Solid Edge part; units mm, degrees
sketch "Sketch1" plane through (0, 0, 0) normal (0, 0, 1) x (1, 0, 0)
  line L0 (-15, 5.75) -> (15, 5.75)
  line L1 (15, 5.75) -> (15, -5.75)
  line L2 (15, -5.75) -> (-15, -5.75)
  line L3 (-15, -5.75) -> (-15, 5.75)
  dimension "D1" = 15
  dimension "D2" = 15
extrude "Protrusion1" add sketch "Sketch1" along normal blind 3
fillet "Avrundningar_1" radius 1 4 edges at (-15, -5.75, 1.5) (15, -5.75, 1.5) (15, 5.75, 1.5) (-15, 5.75, 1.5)
sketch "Sketch2" plane through (0, 0, 3) normal (0, 0, 1) x (0, 1, 0)
  circle A0 centre (-2.75, 12) radius 1.5598
  circle A1 centre (2.75, 12) radius 1.5598
  circle A2 centre (-2.75, -12) radius 1.5598
  circle A3 centre (2.75, -12) radius 1.5598
  dimension "D1" = 2.75
  dimension "D2" = 2.75
extrude "Försänkningar_för_fjäder" cut sketch "Sketch2" against normal blind 1
Part model, mm, in its own coordinate system. A direction names the side the tool comes from. Coordinates: 2 decimals unless noted, no trailing zeros. Write each loop counter-clockwise with the first axis right and the second up, starting at its lowest first coordinate (ties: lowest second). Pieces come first, ordered by that corner, then holes.
Item 1: Pin check, flat tips, straight feed: pin 1 (1.9 mm diameter, centred on x = -12, y = 2.75, fed in from -Z); pin 2 (2.5 mm diameter, centred on x = -12, y = -2.75, fed in from +Z). Stop position of each tip, or through.
Item 2: Probe line 1 (Y direction, x = 12, z = 2.35); line 2 (X direction, y = 2.75, z = 2.35); line 3 (X direction, y = 2.5, z = 2.1). List the from-to ranges inside material, lowest first.
Item 3: Slice it at A-A (y = 2.75). Write the cut outline in (x, z).
Item 4: Mould opens along X. For faces 1 (the face through (14.715, 5.449, 1.521)), 2 (the face through (-14.715, -5.449, 1.521)), 3 (the face through (0, -5.75, 1)), 4 (the face through (12, 3, 2)) say: released by +X, released by -X, zero draft, split by the parting line, or undercut.
Item 5: Which spindle directions (+Z, -Z, +X, -X, +Y, -Y) get a long thin tool onto all of the face, cutting with end or side? Do faces 5 (the face through (-12, -3, 2)), 6 (the face through (0, 0, 3)). Say none if no direction does.
Item 6: Slice it at B-B (x = 12). Write the cut outline in (y, z).
Results found:
1. pin 1: stops at z = 0
1. pin 2: stops at z = 2
2. line 1: y = -5.75 to -4.31, -1.19 to 1.19, 4.31 to 5.75
2. line 2: x = -15 to -13.56, -10.44 to 10.44, 13.56 to 15
2. line 3: x = -15 to -13.54, -10.46 to 10.46, 13.54 to 15
3. outline: (-15, 0) - (15, 0) - (15, 3) - (13.56, 3) - (13.56, 2) - (10.44, 2) - (10.44, 3) - (-10.44, 3) - (-10.44, 2) - (-13.56, 2) - (-13.56, 3) - (-15, 3) - close
4. face 1: released by +X
4. face 2: released by -X
4. face 3: zero draft
4. face 4: undercut
5. face 5: +Z
5. face 6: +Z, +X, -X, +Y, -Y
6. outline: (-5.75, 0) - (5.75, 0) - (5.75, 3) - (4.31, 3) - (4.31, 2) - (1.19, 2) - (1.19, 3) - (-1.19, 3) - (-1.19, 2) - (-4.31, 2) - (-4.31, 3) - (-5.75, 3) - close
